Could you check a few things on this drawing? It's one solid part, dimensions in mm from its lowest x, y, z. A direction names the side the tool comes from. Give positions to 0.01 mm unless a question says otherwise; leave off trailing zeros. Loops run counter-clockwise (first coordinate to the right, second up) from the corner with the lowest first, then second, coordinate; pieces in that order, holes last.
Q1. I'm going to push flat-ended pins straight in: P1, Ø10, axis at y = 18.5, z = 23.5, coming from the +X side; P2, Ø11.5, axis at x = 46.5, z = 6, coming from the +Y side; P3, Ø4, axis at x = 90, y = 27, coming from the +Z side; P4, Ø1.5, axis at x = 18, y = 14.5, coming from the -Z side. Where does each tip first touch, or does it pass through?
Q2. Suppose I cut it at B-B (x = 137.25). List the corners of the cut face in (y, z) for me, and give its area (4 significant figures).
Q3. I need wall thicknesses on probe 1 along Z at (x, y) = (96.45, 0.4); probe 2 along Z at (x, y) = (31, 25.75); probe 3 along Y at (x, z) = (112.5, 19.5). Which ranges of each line are inside material? Lowest first, please.
Q4. Suppose I cut it at A-A (z = 7.5). List the corners of the cut face in (x, y) for me, and give its area (3 significant figures).
Q5. Suppose I cut it at D-D (y = 11). List the corners of the cut face in (x, z) for me.
Q6. Suppose I cut it at C-C (x = 107). List the corners of the cut face in (y, z) for me.
Q7. For the marked faces 1, 2 and 3, which set-ups out of +Z, -Z, +X, -X, +Y, -Y let a thin tool reach every point of the face, with its end or its side?
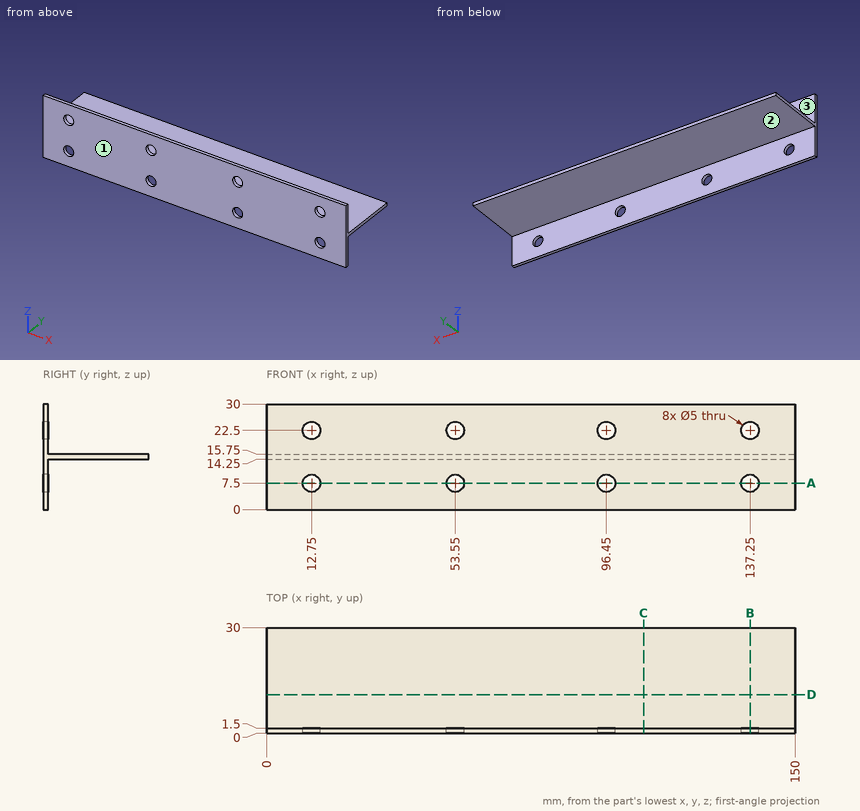
Solutions:
1. P1: passes through
1. P2: stops at y = 1.5
1. P3: stops at z = 15.75
1. P4: stops at z = 14.25
2. outline: (0, 0) - (1.5, 0) - (1.5, 5) - (0, 5) - close; (0, 10) - (1.5, 10) - (1.5, 14.25) - (30, 14.25) - (30, 15.75) - (1.5, 15.75) - (1.5, 20) - (0, 20) - close; (0, 25) - (1.5, 25) - (1.5, 30) - (0, 30) - close
2. area: 72.75 mm2
3. probe 1: z = 0 to 5, 10 to 20, 25 to 30
3. probe 2: z = 14.25 to 15.75
3. probe 3: y = 0 to 1.5
4. outline: (0, 0) - (10.25, 0) - (10.25, 1.5) - (0, 1.5) - close; (15.25, 0) - (51.05, 0) - (51.05, 1.5) - (15.25, 1.5) - close; (56.05, 0) - (93.95, 0) - (93.95, 1.5) - (56.05, 1.5) - close; (98.95, 0) - (134.75, 0) - (134.75, 1.5) - (98.95, 1.5) - close; (139.75, 0) - (150, 0) - (150, 1.5) - (139.75, 1.5) - close
4. area: 195 mm2
5. outline: (0, 14.25) - (150, 14.25) - (150, 15.75) - (0, 15.75) - close
6. outline: (0, 0) - (1.5, 0) - (1.5, 14.25) - (30, 14.25) - (30, 15.75) - (1.5, 15.75) - (1.5, 30) - (0, 30) - close
7. face 1: +Z, -Z, +X, -X, -Y
7. face 2: -Z, +X, -X, +Y
7. face 3: +Z, +X, -X, +Y
